Print and shaded views of the part. All mm, measured from the part's lowest x, y and z. A direction names the side the tool comes from. Round coordinates to 2 decimals unless told otherwise and drop trailing zeros. Order: outer loops, then holes, each group sorted by start corner. A loop starts at its lowest first (then second) coordinate and runs counter-clockwise, first axis right, second up. Notation, with made-up numbers: (84, -39.5) -> (130, -39.5) arc R23 cw to (130, -16.5) -> close; hole circle Ø10 at (70, 62). An arc over 180 degrees is marked (long way). Answer as CSV lines item,"result". Start each with the question number.
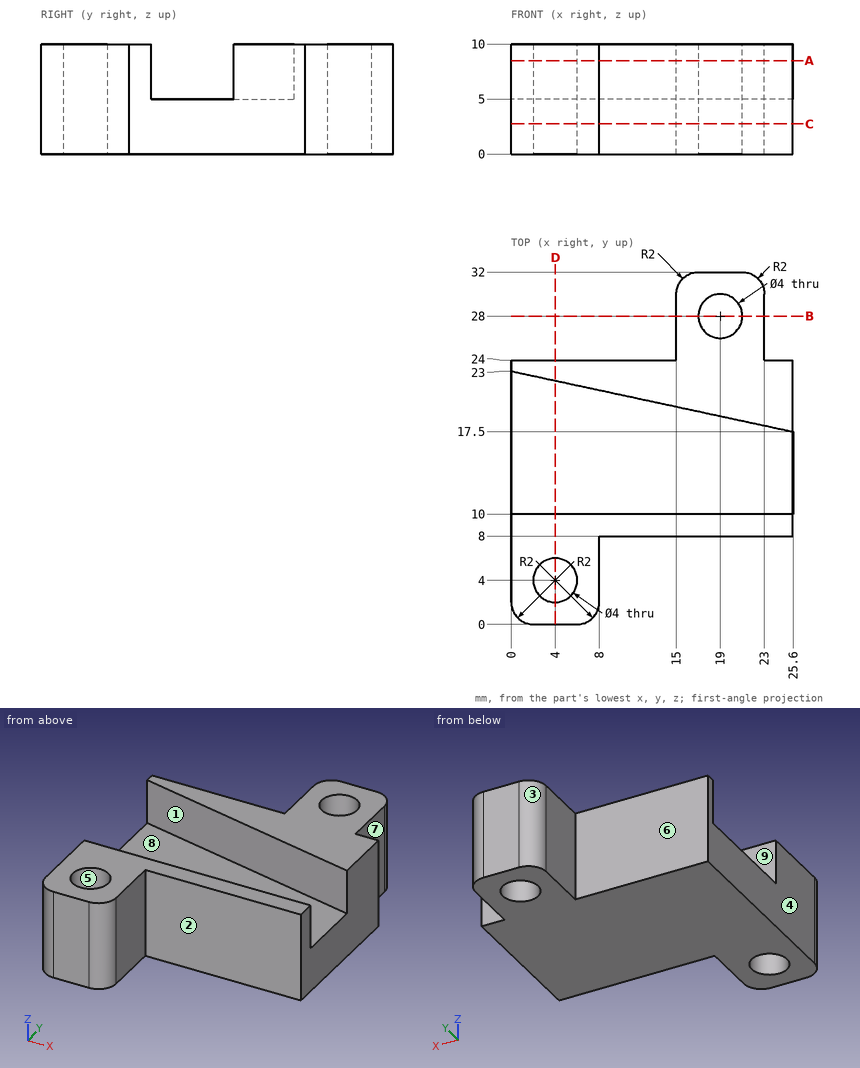
Item 1: Band-saw the part on D-D, the plane x = 4. Give the cut face in (y, z).
Item 2: Band-saw the part on B-B, the plane y = 28. Give the cut face in (x, z), and give its area (3 significant figures).
Item 3: Probe line 1 (Y direction, x = 4, z = 3); line 2 (Y direction, x = 4, z = 6.25); line 3 (Y direction, x = 19, z = 7.25). List the from-to ranges inside material, lowest first.
Item 4: Tool access for the marked faces 5, 6, 7, 8 and 9: list every direction of +Z, -Z, +X, -X, +Y, -Y with a clear straight run to the whole face (end or side of a thin tool).
Item 5: Mould opens along Y. For the marked faces 1, 2, 3 and 4 say: released by +Y, released by -Y, zero draft, split by the parting line, or undercut.
Item 6: Band-saw the part on A-A, the plane z = 8.5. Give the cut face in (x, y).
Item 7: Band-saw the part on C-C, the plane z = 2.75. Give the cut face in (x, y), and give its area (3 significant figures).
Item 8: Pin check, flat tips, straight feed: pin 1 (3 mm diameter, centred on x = 7.5, z = 2, fed in from +Y); pin 2 (3 mm diameter, centred on x = 19, y = 28, fed in from -Z); pin 3 (4 mm diameter, centred on x = 17.5, y = 15, fed in from +Z); pin 4 (1.8 mm diameter, centred on y = 27.5, z = 6.5, fed in from +X). Stop position of each tip, or through.
Values:
1,outline,"(0, 0) -> (2, 0) -> (2, 10) -> (0, 10) -> close; (6, 0) -> (24, 0) -> (24, 10) -> (22.14, 10) -> (22.14, 5) -> (10, 5) -> (10, 10) -> (6, 10) -> close"
2,outline,"(15, 0) -> (17, 0) -> (17, 10) -> (15, 10) -> close; (21, 0) -> (23, 0) -> (23, 10) -> (21, 10) -> close"
2,area,"40.0 mm²"
3,line 1,"0 to 2, 6 to 24"
3,line 2,"0 to 2, 6 to 10, 22.14 to 24"
3,line 3,"8 to 10, 18.92 to 26, 30 to 32"
4,face 5,"+Z, -Z"
4,face 6,"+Z, -Z, -X, +Y"
4,face 7,"+Z, -Z, +X, +Y"
4,face 8,"+Z, -X"
4,face 9,"+Z, +X, -X"
5,face 1,"undercut"
5,face 2,"released by -Y"
5,face 3,"released by +Y"
5,face 4,"zero draft"
6,outline,"(0, 2) arc R2 ccw to (2, 0) -> (6, 0) arc R2 ccw to (8, 2) -> (8, 8) -> (25.6, 8) -> (25.6, 10) -> (0, 10) -> close; (0, 23) -> (25.6, 17.5) -> (25.6, 24) -> (23, 24) -> (23, 30) arc R2 ccw to (21, 32) -> (17, 32) arc R2 ccw to (15, 30) -> (15, 24) -> (0, 24) -> close; hole circle Ø4 at (4, 4); hole circle Ø4 at (19, 28)"
7,outline,"(0, 2) arc R2 ccw to (2, 0) -> (6, 0) arc R2 ccw to (8, 2) -> (8, 8) -> (25.6, 8) -> (25.6, 24) -> (23, 24) -> (23, 30) arc R2 ccw to (21, 32) -> (17, 32) arc R2 ccw to (15, 30) -> (15, 24) -> (0, 24) -> close; hole circle Ø4 at (4, 4); hole circle Ø4 at (19, 28)"
7,area,"509 mm²"
8,pin 1,"y = 24"
8,pin 2,"through"
8,pin 3,"z = 5"
8,pin 4,"x = 23"
